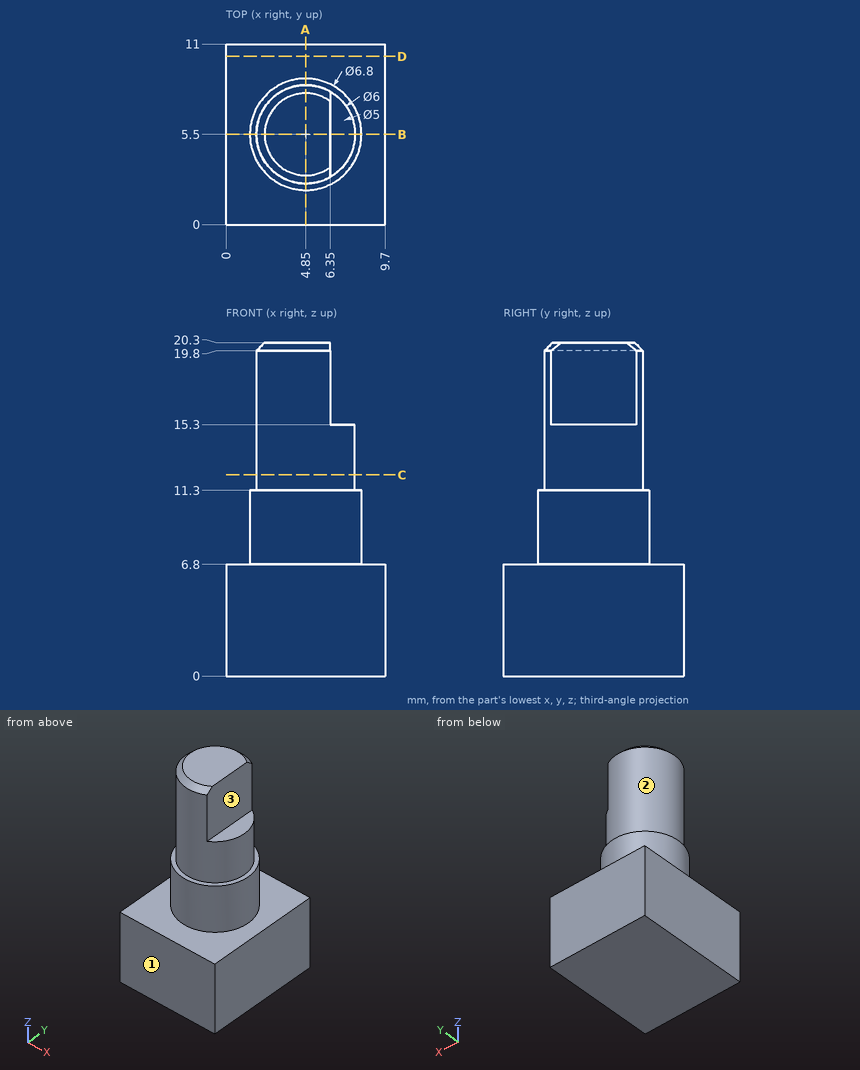
Can you work these out from the drawing? Everything is in mm from the part's minimum corner. A direction names the side the tool comes from. Coordinates: 2 decimals unless noted, no trailing zeros. Loops run counter-clockwise (first coordinate to the right, second up) from the corner with the lowest first, then second, coordinate; pieces in that order, holes last. Notation, with made-up numbers: M 68.25,54 L 78.25,54 A21 cw 78.25,66 Z; hole C 72,-31.75 d6. An arc over 180 degrees is marked long. Put each result on its own line as item: value. Start each with the question number.
(1) Suppose I cut it at B-B on y = 5.5. Please give me the cut outline in (x, z), then the cut area to 3 significant figures.
(2) Will these pins go through, and if not, where does the flat tip stop? P1, Ø2.5, axis at y = 4.5, z = 17, coming from the +X side; P2, Ø1.5, axis at x = 5.5, z = 9, coming from the -Y side; P3, Ø4, axis at x = 6, z = 17, coming from the -Y side.
(3) For the marked faces 1, 2 and 3, which set-ups out of +Z, -Z, +X, -X, +Y, -Y let a thin tool reach every point of the face, with its end or its side?
(4) Suppose I cut it at C-C on z = 12.25. Please give me the cut outline in (x, y).
(5) Suppose I cut it at A-A on x = 4.85. Please give me the cut outline in (y, z).
(6) Suppose I cut it at D-D on y = 10.25. Please give me the cut outline in (x, z).
(7) I need wall thicknesses on line 1 (Z direction, x = 2.5, y = 1.25); line 2 (Z direction, x = 7, y = 6); line 3 (X direction, y = 3.75, z = 8). Which ranges of each line are inside material? Lowest first, please. Write a range as from..to.
Solutions:
1. outline: M 0,0 L 9.7,0 L 9.7,6.8 L 8.25,6.8 L 8.25,11.3 L 7.85,11.3 L 7.85,15.3 L 6.35,15.3 L 6.35,20.3 L 2.35,20.3 L 1.85,19.8 L 1.85,11.3 L 1.45,11.3 L 1.45,6.8 L 0,6.8 Z
1. area: 143 mm2
2. P1: stops at x = 6.35
2. P2: stops at y = 2.1
2. P3: stops at y = 2.5
3. face 1: +Z, -Z, +X, -X, -Y
3. face 2: +Z
3. face 3: +Z, +X, +Y, -Y
4. outline: C 4.85,5.5 d6
5. outline: M 0,0 L 11,0 L 11,6.8 L 8.9,6.8 L 8.9,11.3 L 8.5,11.3 L 8.5,19.8 L 8,20.3 L 3,20.3 L 2.5,19.8 L 2.5,11.3 L 2.1,11.3 L 2.1,6.8 L 0,6.8 Z
6. outline: M 0,0 L 9.7,0 L 9.7,6.8 L 0,6.8 Z
7. line 1: z = 0..6.8
7. line 2: z = 0..15.3
7. line 3: x = 1.93..7.77
